Work out the finished part from the listing and answer in its coordinate system (mm). A direction names the side the tool comes from. Give positions to 0.01 mm unless a question says otherwise; leave off trailing zeros. Write each loop counter-clockwise with the first axis right and the second up, starting at its lowest first coordinate (ties: lowest second). Pieces come first, ordered by that corner, then holes.
1) Straight lines are drawn through the part: probe 1 along X at (y, z) = (-30.5, 12); probe 2 along Z at (x, y) = (4.95, 33); probe 3 along Z at (x, y) = (1, 11). For each, find the intervals that lie inside material, in ascending order.
2) Find section B-B (z = 9.5). Determine the outline of the cut face in (x, y), plus the area to 3 significant figures.
3) Given pin 1 Ø3 at (x, y) = (15.5, -13) entering from +Z; pin 2 Ø12 at (y, z) = (-12, 18) entering from -X; pin 3 Ø2 at (x, z) = (-5.5, 26) entering from -Y, each flat-ended and moving along its own axis, determine where each tip first touches the part or whether it passes through.
4) A tool of negligible diameter and unlimited length cuts with its end or side. For faces 4 (the face through (-15, -1, 3)), 5 (the face through (-4, -1, 18)), 6 (the face through (-5, 40, 8)), from which of +Z, -Z, +X, -X, +Y, -Y can it reach the whole face along a straight path? Write none if from no direction.
5) Find section A-A (z = 17). Determine the outline of the cut face in (x, y).
6) Determine the mould class of faces 1 (the face through (16.07, -38.5, 1.52)), 2 (the face through (5.5, 31.5, 18.4)), 3 (the face through (0, -1, 3)) for opening direction Z: pulls with the +Z half, pulls with the -Z half, needs draft (parallel to the pull), parting line crosses it, or undercut.
7) Find section C-C (y = -22.5). Determine the outline of the cut face in (x, z), plus the area to 3 significant figures.
8) Find section D-D (y = 33). Determine the outline of the cut face in (x, z), plus the area to 3 significant figures.
```python
from build123d import *

# Parameters (mm, degrees)
F1_DEPTH = 40
F2_R     = 2
F3_R     = 10
F4_R     = 2.05
F5_DEPTH = 14
F6_R     = 5
F7_R     = 5


with BuildPart() as f1:
    # F0 (on Front) → F1 (new body, symmetric)
    with BuildSketch(Plane.XZ):
        Polygon((-17.5, 3), (-17.5, 0), (17.5, 0), (17.5, 3), (7, 3), (7, 32), (4, 32), (4, 3), (-4, 3), (-4, 32), (-7, 32), (-7, 3), align=None)
    extrude(amount=F1_DEPTH, both=True)

    # F2
    f2_edges = [f1.edges().sort_by_distance(p)[0] for p in [
        (-4, 0, 3),
        (4, 0, 3),
    ]]
    fillet(f2_edges, radius=F2_R)

    # F3
    f3_edges = [f1.edges().sort_by_distance(p)[0] for p in [
        (5.5, 40, 32),
        (-5.5, 40, 32),
        (5.5, -40, 32),
        (-5.5, -40, 32),
    ]]
    fillet(f3_edges, radius=F3_R)

    # F4 (on face) → F5 (cut, through all)
    with BuildSketch(Plane.YZ.offset(7)):
        with Locations((-33, 17)):
            Circle(F4_R)
        with Locations((33, 17)):
            Circle(F4_R)
    extrude(amount=-F5_DEPTH, mode=Mode.SUBTRACT)

    # F6
    f6_edges = [f1.edges().sort_by_distance(p)[0] for p in [
        (7, 0, 3),
        (-7, 0, 3),
    ]]
    fillet(f6_edges, radius=F6_R)

    # F7
    f7_edges = [f1.edges().sort_by_distance(p)[0] for p in [
        (-17.5, -40, 1.5),
        (17.5, -40, 1.5),
        (17.5, 40, 1.5),
        (-17.5, 40, 1.5),
    ]]
    fillet(f7_edges, radius=F7_R)


solid = f1.part
```
Results:
1. probe 1: x = -7 to -4, 4 to 7
1. probe 2: z = 0 to 14.95, 19.05 to 31.54
1. probe 3: z = 0 to 3
2. outline: (-7, -40) - (-4, -40) - (-4, 40) - (-7, 40) - close; (4, -40) - (7, -40) - (7, 40) - (4, 40) - close
2. area: 480 mm2
3. pin 1: stops at z = 3
3. pin 2: stops at x = -7
3. pin 3: stops at y = -39.54
4. face 4: +Z, -X, +Y, -Y
4. face 5: +Z, +Y, -Y
4. face 6: +Z, -Z, +X, -X, +Y
5. outline: (-7, -40) - (-4, -40) - (-4, -35.05) - (-7, -35.05) - close; (-7, -30.95) - (-4, -30.95) - (-4, 30.95) - (-7, 30.95) - close; (-7, 35.05) - (-4, 35.05) - (-4, 40) - (-7, 40) - close; (4, -40) - (7, -40) - (7, -35.05) - (4, -35.05) - close; (4, -30.95) - (7, -30.95) - (7, 30.95) - (4, 30.95) - close; (4, 35.05) - (7, 35.05) - (7, 40) - (4, 40) - close
6. face 1: needs draft
6. face 2: undercut
6. face 3: pulls with the +Z half
7. outline: (-17.5, 0) - (17.5, 0) - (17.5, 3) - (12, 3) arc R5 cw to (7, 8) - (7, 32) - (4, 32) - (4, 5) arc R2 cw to (2, 3) - (-2, 3) arc R2 cw to (-4, 5) - (-4, 32) - (-7, 32) - (-7, 8) arc R5 cw to (-12, 3) - (-17.5, 3) - close
7. area: 291 mm2
8. outline: (-17.5, 0) - (17.5, 0) - (17.5, 3) - (12, 3) arc R5 cw to (7, 8) - (7, 14.95) - (4, 14.95) - (4, 5) arc R2 cw to (2, 3) - (-2, 3) arc R2 cw to (-4, 5) - (-4, 14.95) - (-7, 14.95) - (-7, 8) arc R5 cw to (-12, 3) - (-17.5, 3) - close; (-7, 19.05) - (-4, 19.05) - (-4, 31.54) - (-7, 31.54) - close; (4, 19.05) - (7, 19.05) - (7, 31.54) - (4, 31.54) - close
8. area: 264 mm2
